Input: part model. Units: mm. Frame: model coordinates. A direction names the side the tool comes from. Coordinates: 2 decimals unless noted, no trailing zeros. Write each loop counter-clockwise with the first axis right and the second up, starting at its lowest first coordinate (ties: lowest second). Pieces come first, ordered by that corner, then holes. Notation, with made-up numbers: M 8,52 L 45,52 A17 ccw 45,65 Z; hole C 43.5,-28.5 d3. An arc over 180 degrees is marked long. Answer as a JSON object with one key per item and string values. Group by question number.
from build123d import *

# Parameters (mm, degrees)
SKETCH1_W           = 1.5875
SKETCH1_H           = 3.109195134
SKETCH1_H_2         = 3.240804866
BOSS_EXTRUDE1_DEPTH = 1.5875


with BuildPart() as part:
    # Sketch1 → Boss-Extrude1 (new body)
    with BuildSketch(Plane(origin=(0, 0, 0), x_dir=(0, 0, -1), z_dir=(1, 0, 0))):
        with BuildLine():
            ThreePointArc((-23.848326893, -26.661593728), (-20.937975975, -10.862409095), (-35.836269612, -4.8519828))
            Line((-35.836269612, -4.8519828), (0, 6.284195134))
            Line((0, 6.284195134), (0, -6.415804866))
            Line((0, -6.415804866), (-23.848326893, -26.661593728))
        make_face()
        with Locations((0.79375, 4.729597567)):
            Rectangle(SKETCH1_W, SKETCH1_H)
        with Locations((0.79375, -4.795402433)):
            Rectangle(SKETCH1_W, SKETCH1_H_2)
        Polygon((-4.845708228, -12.611927822), (-5.873104867, -11.401716106), (-17.975222027, -21.675682489), (-16.947825388, -22.885894205), align=None)
    extrude(amount=BOSS_EXTRUDE1_DEPTH)


solid = part.part
Q1. Section C-C, the plane y = -24. Return the cut outline in (x, z).
Q2. Section B-B, the plane z = 15. Return the cut outline in (x, y), and give its area (3 significant figures).
Q3. Pin query (flat end, axial travel): pin 1 Ø0.8 at (x, z) = (0.5, -0.5) entering from -Y; pin 2 Ø0.5 at (x, y) = (1, -1.5) entering from -Z. Return the tip coordinate at first contact, or that it passes through.
Q4. Line query: line 1 (Y direction, x = 0.95, z = 21.5); line 2 (Y direction, x = 0.55, z = 11); line 3 (Z direction, x = 0.2, y = -19.5). Output: solid intervals per line, ascending. Write a range as from..to.
Q5. Draft query along Y for faces 1 (the flat face through (1, 0, 0)), 2 (the flat face through (0.783, -24.134, 20.871)), 3 (the cylindrical face through (0.78, -11.08, 20.82)), 4 (the flat face through (1, -5, -1.588)). Return one class per face: released by +Y, released by -Y, zero draft, split by the parting line, or undercut.
Q6. Access query for faces 5 (the flat face through (0, -6, 13)), 6 (the flat face through (1, -6.416, -1)), 7 (the flat face through (1.588, -6, 13)), 8 (the flat face through (1, 3.175, -1)), 9 (the flat face through (0.78, -22.27, 17.47)). Directions: +Z, -Z, +X, -X, +Y, -Y. A direction counts if a zero-diameter tool reaches every point of the face in a straight line with its end or side. Return the directions, or none.
Q7. Section A-A, the plane x = 0.65. Return the cut outline in (y, z) (1 decimal), and give its area (3 significant figures).
Filled in:
{
 "1": {"outline": "M 0,20.71 L 1.59,20.71 L 1.59,21.48 L 0,21.48 Z"},
 "2": {"outline": "M 0,-21.23 L 1.59,-21.23 L 1.59,1.62 L 0,1.62 Z", "area": "36.3 mm^2"},
 "3": {"pin 1": "y = -6.42", "pin 2": "z = 0"},
 "4": {"line 1": "-24.67..-24.02, -9.94..-0.4", "line 2": "-17.84..2.87", "line 3": "12.96..19.62"},
 "5": {"face 1": "undercut", "face 2": "released by -Y", "face 3": "undercut", "face 4": "zero draft"},
 "6": {"face 5": "+Z, -Z, -X, +Y, -Y", "face 6": "-Z, +X, -X, -Y", "face 7": "+Z, -Z, +X, +Y, -Y", "face 8": "-Z, +X, -X", "face 9": "+X, -X, -Y"},
 "7": {"outline": "M -26.7,23.8 L -21.7,18 L -22.9,16.9 L -12.6,4.8 L -11.4,5.9 L -6.4,0 L -6.4,-1.6 L -3.2,-1.6 L -3.2,0 L 3.2,0 L 3.2,-1.6 L 6.3,-1.6 L 6.3,0 L -4.9,35.8 A12.7 cw Z", "area": "455 mm^2"}
}
